Could you check a few things on this model? Use its own coordinates, in mm. Face numbers are marked on the shaded views. A direction names the side the tool comes from. Give positions to 0.01 mm unless a question says otherwise; leave off trailing zeros. Loops run counter-clockwise (first coordinate to the right, second up) from the corner with the lowest first, then second, coordinate; pieces in that order, holes last. Notation, with made-up numbers: M -25.5,31.5 L -6.5,31.5 A10 cw -6.5,35.5 Z; hole C 14.5,8 d11. An arc over 180 degrees is marked long. Use a Markdown table: item, result. Add a question column.
1) We'd pull the mould along X, two halves only. Please class the marked faces 3, 4, 5 and 6: +X half, -X half, draft (parallel to the pull), parting line (faces both ways), or undercut.
2) Suppose I cut it at C-C on x = -15.75. List the corners of the cut face in (y, z) for me (3 decimals).
3) Suppose I cut it at B-B on y = 78. List the corners of the cut face in (x, z) for me, and give its area (3 significant figures).
4) Which directions (+Z, -Z, +X, -X, +Y, -Y) give clear straight access to the entire face, cutting with the end or side of a thin tool? Please do the marked faces 1 and 2.
5) Suppose I cut it at A-A on x = -7.75. List the corners of the cut face in (y, z) for me (3 decimals), and give its area (3 significant figures).
6) Will these pins go through, and if not, where does the flat tip stop? pin 1 Ø10.5 at (x, z) = (-10.5, 18.5) entering from -Y; pin 2 Ø2 at (x, y) = (-6.5, 75) entering from +Z; pin 3 Ø1 at (x, y) = (-11, 79) entering from +Z.
7) Suppose I cut it at D-D on z = 6.25. List the corners of the cut face in (x, y) for me.
8) If I drill on line 1 along Y through (x, z) = (-7.75, 8.75); line 2 along Y through (x, z) = (-7.5, 20); line 3 along Z through (x, y) = (-4, 74.5), over which ranges is the centre line in solid material (lowest first)? Write a range as [from, to].
Autodesk Inventor part; units mm, degrees
ref_plane "YZ Plane" through (0, 0, 0) normal (1, 0, 0) x (0, 1, 0)
ref_plane "XZ Plane" through (0, 0, 0) normal (0, 1, 0) x (-1, 0, 0)
ref_plane "XY Plane" through (0, 0, 0) normal (0, 0, 1) x (1, 0, 0)
ref_plane "Work Plane1" through (0, 0, 0) normal (0, 0, 1) x (1, 0, 0)
sketch "Sketch1" plane through (0, 0, 0) normal (0, 0, 1) x (1, 0, 0)
  line L0 (17.75, 85) -> (-18.004, 85) construction
  circle A0 centre (-7.75, 70) radius 1.7 construction
  line L1 (-9.375, 72.8146) -> (-6.125, 72.8146) construction
  line L2 (-18.004, 85) -> (-18.004, -85) construction
  line L3 (-3.25, 73.1895) -> (-3.25, 76.1105) construction
  line L4 (-11, 70) -> (-9.375, 72.8146) construction
  line L5 (3.2502, 74.65) -> (3.2502, 77.444) construction
  line L6 (3.2502, 77.825) -> (3.2502, 81) construction
  line L7 (-0.127, 85) -> (-18.004, 85)
  line L8 (-18.004, 85) -> (-18.004, 72.8146)
  line L9 (-18.004, 72.8146) -> (-0.127, 72.8146)
  line L10 (-0.127, 72.8146) -> (-0.127, 85)
  circle A1 centre (-7.75, 76.8764) radius 1.7
  point P0 (0, 0)
  dimension "d0" = 3.4
  dimension "d1" = 12.1854
  dimension "d3" = 17.877
  dimension "d6" = 4.0618
extrude "Leg" add sketch "Sketch1" along normal blind 10
sketch "Sketch2" plane through (0, 0, 10) normal (0, 0, 1) x (1, 0, 0)
  line L0 (-0.127, 72.8146) -> (-0.127, 85)
  line L1 (-18.004, 85) -> (-18.004, 72.8146)
  line L2 (-18.004, 85) -> (-18.004, 80.9625)
  line L3 (-0.127, 80.9625) -> (-0.127, 85)
  line L4 (-0.127, 85) -> (-18.004, 85)
  line L5 (-18.004, 85) -> (-18.004, 79.92)
  line L6 (-18.004, 79.92) -> (-0.127, 79.92)
  line L7 (-0.127, 79.92) -> (-0.127, 85)
  point P0 (0, 0)
  dimension "d7" = 5.08
extrude "Extrusion2" add sketch "Sketch2" along normal blind 16
fillet "Fillet1" radius 3.175 1 edges at (-9.0655, 79.92, 10)
equation "\"d6\" = 0.333333 * d1"
properties part number "Mounting Bracket Bottom"
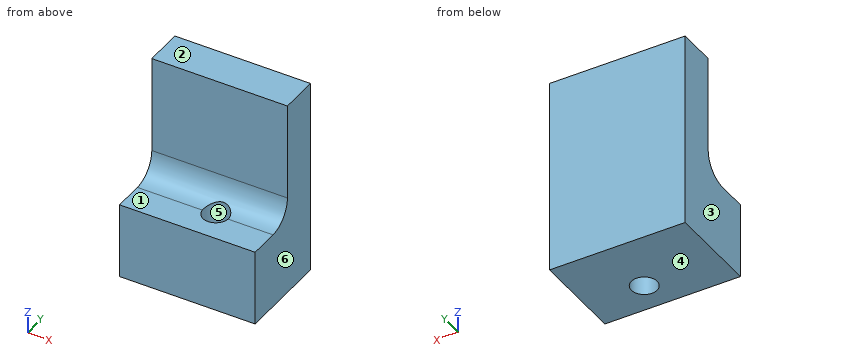
Answer block:
| question | item | result |
|---|---|---|
| 1 | face 3 | -X half |
| 1 | face 4 | draft |
| 1 | face 5 | undercut |
| 1 | face 6 | +X half |
| 2 | outline | M 72.815,0 L 85,0 L 85,26 L 79.92,26 L 79.92,13.175 A3.175 cw 76.745,10 L 72.815,10 Z |
| 3 | outline | M -18,0 L -9.03,0 L -9.03,10.26 L -18,10.26 Z; M -6.47,0 L -0.13,0 L -0.13,10.26 L -6.47,10.26 Z |
| 3 | area | 157 mm^2 |
| 4 | face 1 | +Z, +X, -X, -Y |
| 4 | face 2 | +Z, +X, -X, +Y, -Y |
| 5 | outline | M 72.815,0 L 75.176,0 L 75.176,10 L 72.815,10 Z; M 78.576,0 L 85,0 L 85,26 L 79.92,26 L 79.92,13.175 A3.175 cw 78.576,10.581 Z |
| 5 | area | 171 mm^2 |
| 6 | pin 1 | stops at y = 79.92 |
| 6 | pin 2 | stops at z = 10 |
| 6 | pin 3 | stops at z = 11.6 |
| 7 | outline | M -18,72.81 L -0.13,72.81 L -0.13,85 L -18,85 Z; hole C -7.75,76.88 d3.4 |
| 8 | line 1 | y = [72.81, 75.18], [78.58, 85] |
| 8 | line 2 | y = [79.92, 85] |
| 8 | line 3 | z = [0, 10] |
